For this review, take the finished solid that the model builds, in its own axes (mm). Face numbers are marked on the shaded views. A direction names the side the tool comes from. Round coordinates to 2 decimals unless told otherwise and drop trailing zeros. Loops run counter-clockwise (first coordinate to the right, second up) from the corner with the lowest first, then second, coordinate; pieces in that order, holes last.
1) Insertion check: pin 1 (17 mm diameter, centred on y = 10, z = -16.5, fed in from -X); pin 2 (17 mm diameter, centred on y = 24, z = -26.5, fed in from +X); pin 3 (1.2 mm diameter, centred on x = 17, z = 14, fed in from +Y). Each pin has a flat end and moves straight along its axis. Give the tip position at first contact, or say it passes through.
2) Take a section at A-A (y = 34). State the section outline as (x, z) points.
3) Take a section at D-D (x = -2). State the section outline as (y, z) points.
4) Take a section at C-C (z = -20.5). State the section outline as (x, y) points.
5) Wall thickness on L1, parallel to X at y = 21.5, z = 1.5; L2, parallel to Y at x = 26.5, z = -12; L3, parallel to Y at x = -9.5, z = -28: over which ranges is each line inside the solid? List them lowest first.
6) Mouldability with a two-part tool opening along X and no side actions: class the marked faces 4, 5, 6 and 7 as pulls with the +X half, pulls with the -X half, needs draft (parallel to the pull), parting line crosses it, or undercut.
7) Tool access review of the marked faces 1, 2 and 3: name each direction out of +Z, -Z, +X, -X, +Y, -Y from which nothing blocks a thin tool from reaching the whole face with its end or side.
8) Take a section at B-B (x = 31). State the section outline as (y, z) points.
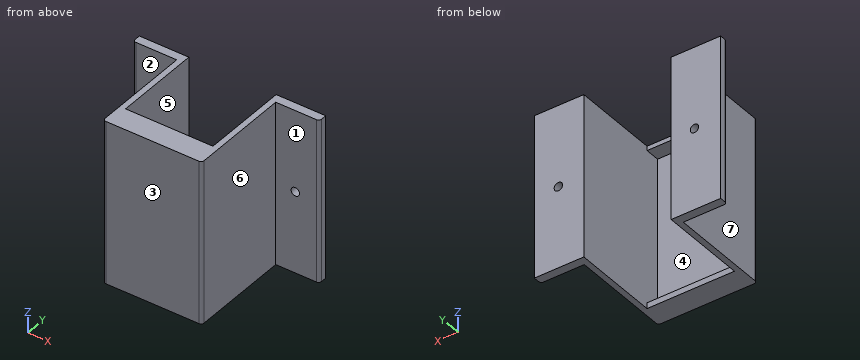
```python
from build123d import *

# Parameters (mm, degrees)
SKETCH2_W           = 34
SKETCH2_H           = 56
BOSS_EXTRUDE1_DEPTH = 3
SKETCH3_W           = 2
SKETCH3_H           = 56
BOSS_EXTRUDE2_DEPTH = 35
SKETCH4_W           = 56
SKETCH4_H           = 2.991859995
BOSS_EXTRUDE3_DEPTH = 15
SKETCH5_W           = 56
SKETCH5_H           = 2.991859995
BOSS_EXTRUDE4_DEPTH = 15
SKETCH6_W           = 30
SKETCH6_H           = 2
SKETCH6_H_2         = 1.5
BOSS_EXTRUDE5_DEPTH = 5
SKETCH8_R           = 1.45
CUT_EXTRUDE1_DEPTH  = 75.275058866
FILLET1_R           = 1


with BuildPart() as part:
    # Sketch2 → Boss-Extrude1 (new body)
    with BuildSketch(Plane(origin=(0, 0, 0), x_dir=(1, 0, 0), z_dir=(0, 1, 0))):
        with Locations((17, 12.887459807)):
            Rectangle(SKETCH2_W, SKETCH2_H)
    extrude(amount=BOSS_EXTRUDE1_DEPTH)

    # Sketch3 → Boss-Extrude2 (add)
    with BuildSketch(Plane(origin=(0, 3, 0), x_dir=(1, 0, 0), z_dir=(0, 1, 0))):
        with Locations((1, 12.887459807)):
            Rectangle(SKETCH3_W, SKETCH3_H)
        with Locations((33, 12.887459807)):
            Rectangle(SKETCH3_W, SKETCH3_H)
    extrude(amount=BOSS_EXTRUDE2_DEPTH)

    # Sketch4 → Boss-Extrude3 (add)
    with BuildSketch(Plane(origin=(34, 0, 0), x_dir=(0, 0, -1), z_dir=(1, 0, 0))):
        with Locations((12.887459807, 36.504070003)):
            Rectangle(SKETCH4_W, SKETCH4_H)
    extrude(amount=BOSS_EXTRUDE3_DEPTH)

    # Sketch5 → Boss-Extrude4 (add)
    with BuildSketch(Plane.ZY):
        with Locations((-12.887459807, 36.504070003)):
            Rectangle(SKETCH5_W, SKETCH5_H)
    extrude(amount=BOSS_EXTRUDE4_DEPTH)

    # Sketch6 → Boss-Extrude5 (add)
    with BuildSketch(Plane(origin=(0, 3, 0), x_dir=(1, 0, 0), z_dir=(0, 1, 0))):
        with Locations((17, 39.887459807)):
            Rectangle(SKETCH6_W, SKETCH6_H)
        with Locations((17, -14.362540193)):
            Rectangle(SKETCH6_W, SKETCH6_H_2)
    extrude(amount=BOSS_EXTRUDE5_DEPTH)

    # Sketch8 → Cut-Extrude1 (cut, through all)
    with BuildSketch(Plane(origin=(0, 38, 0), x_dir=(1, 0, 0), z_dir=(0, 1, 0))):
        with Locations(Location((-6.002072166, 12.887459807, 0), (0, 0, 270))):
            Circle(SKETCH8_R)
        with Locations(Location((40.730432143, 12.887459807, 0), (0, 0, 270))):
            Circle(SKETCH8_R)
    extrude(amount=-CUT_EXTRUDE1_DEPTH, mode=Mode.SUBTRACT)

    # Fillet1
    fillet1_edges = [part.edges().sort_by_distance(p)[0] for p in [
        (49, 35.008140005, -12.887459807),
        (-15, 35.008140005, -12.887459807),
        (34, 0, -12.887459807),
        (0, 0, -12.887459807),
    ]]
    fillet(fillet1_edges, radius=FILLET1_R)


solid = part.part
```
Response:
1. pin 1: stops at x = 0
1. pin 2: stops at x = 34
1. pin 3: stops at y = 8
2. outline: (0, -40.89) - (2, -40.89) - (2, 15.11) - (0, 15.11) - close; (32, -40.89) - (34, -40.89) - (34, 15.11) - (32, 15.11) - close
3. outline: (35.01, -40.89) - (38, -40.89) - (38, 15.11) - (35.01, 15.11) - close
4. outline: (-15, 36.01) arc R1 ccw to (-14, 35.01) - (0, 35.01) - (0, 1) arc R1 ccw to (1, 0) - (33, 0) arc R1 ccw to (34, 1) - (34, 35.01) - (48, 35.01) arc R1 ccw to (49, 36.01) - (49, 38) - (32, 38) - (32, 3) - (2, 3) - (2, 38) - (-15, 38) - close
5. L1: x = 0 to 2, 32 to 34
5. L2: y = 0 to 3
5. L3: y = 35.01 to 38
6. face 4: undercut
6. face 5: undercut
6. face 6: pulls with the +X half
6. face 7: pulls with the -X half
7. face 1: +Z, -Z, +X, -Y
7. face 2: +Z, -Z, -X, -Y
7. face 3: +Z, -Z, +X, -X, -Y
8. outline: (0, -40.89) - (8, -40.89) - (8, -38.89) - (3, -38.89) - (3, 13.61) - (8, 13.61) - (8, 15.11) - (0, 15.11) - close
